The listing builds one solid part. Answer for the finished solid, in the listing's coordinates (mm). Face numbers are marked on the shaded views. A direction names the side the tool comes from. Coordinates: 2 decimals unless noted, no trailing zeros. Loops run counter-clockwise (first coordinate to the right, second up) from the corner with the lowest first, then second, coordinate; pieces in that order, holes last. Notation, with made-up numbers: (33.5, 7) - (92.5, 7) arc R24 ccw to (92.5, 30) - close; hole circle Ø2 at (-39, 62). An arc over 180 degrees is marked (long way). One line per question, with ' | ' between items.
from build123d import *

# Parameters (mm, degrees)
SKETCH_1_W          = 40
SKETCH_1_H          = 30
EXTRUDE_2_DEPTH     = 6
SKETCH_2_W          = 30
SKETCH_2_H          = 8.15479
EXTRUDE_4_DEPTH     = 30
SKETCH_4_R          = 5
CUT_EXTRUDE_1_DEPTH = 51.950956811
FILLET_1_R          = 10
FILLET_2_R          = 10


with BuildPart() as part:
    # Эскиз1 → Бобышка-Вытянуть2 (new body)
    with BuildSketch(Plane.XY):
        Rectangle(SKETCH_1_W, SKETCH_1_H)
    extrude(amount=EXTRUDE_2_DEPTH)

    # Эскиз2 → Бобышка-Вытянуть4 (add)
    with BuildSketch(Plane.XY.offset(6)):
        with Locations((0, -10.922605)):
            Rectangle(SKETCH_2_W, SKETCH_2_H)
    extrude(amount=EXTRUDE_4_DEPTH)

    # Эскиз4 → Вырез-Вытянуть1 (cut, through all)
    with BuildSketch(Plane(origin=(0, -15, 0), x_dir=(-1, 0, 0), z_dir=(0, -1, 0))):
        with Locations(Location((0, -21, 0), (0, 0, 180))):
            Circle(SKETCH_4_R)
    extrude(amount=-CUT_EXTRUDE_1_DEPTH, mode=Mode.SUBTRACT)

    # Скругление1
    fillet_1_edges = [part.edges().sort_by_distance(p)[0] for p in [
        (-15, -10.922605, 36),
    ]]
    fillet(fillet_1_edges, radius=FILLET_1_R)

    # Скругление2
    fillet_2_edges = [part.edges().sort_by_distance(p)[0] for p in [
        (15, -10.922605, 36),
    ]]
    fillet(fillet_2_edges, radius=FILLET_2_R)


solid = part.part
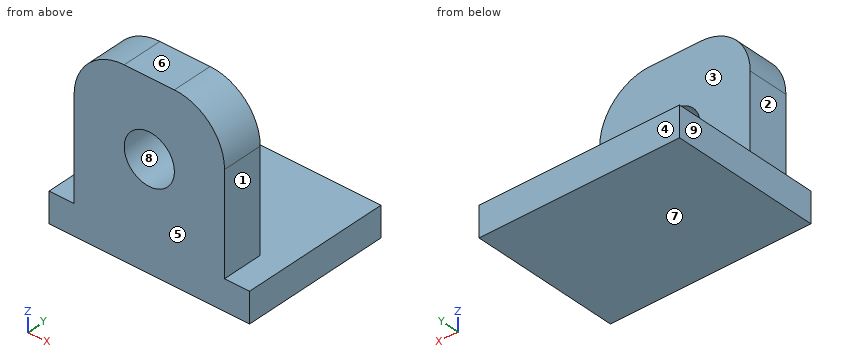
Item 1: Each of these flat-tipped pins is pushed along its axis until it touches: pin 1 Ø4 at (x, z) = (-5, 24.5) entering from +Y; pin 2 Ø3 at (x, y) = (12, 4) entering from +Z; pin 3 Ø9 at (y, z) = (-11.5, 12.5) entering from +X. Where does it stop, or does it pass through?
Taken from the geometry:
pin 1: stops at y = -6.85 | pin 2: stops at z = 6 | pin 3: stops at x = 15
Item 2: The mould has two halves that part along Z. Classify the marked faces 6, 7, 8 and 9: pulls with the +Z half, pulls with the -Z half, needs draft (parallel to the pull), parting line crosses it, or undercut.
Taken from the geometry:
face 6: pulls with the +Z half | face 7: pulls with the -Z half | face 8: undercut | face 9: needs draft
Item 3: Find section A-A, the plane y = -10.5. Write down the section's boundary in (x, z), plus the area to 3 significant figures.
Taken from the geometry:
outline: (-20, 0) - (20, 0) - (20, 6) - (15, 6) - (15, 26) arc R10 ccw to (5, 36) - (-5, 36) arc R10 ccw to (-15, 26) - (-15, 6) - (-20, 6) - close; hole circle Ø10 at (0, 21) | area: 1,020 mm2
Item 4: Find the intervals of material crossed by line 1 (Z direction, x = 0, y = -12); line 2 (Y direction, x = 6, z = 28); line 3 (Z direction, x = 2, y = 6.5), in increasing order. Write a range as [from, to].
Taken from the geometry:
line 1: z = [0, 16], [26, 36] | line 2: y = [-15, -6.85] | line 3: z = [0, 6]
Item 5: Find section D-D, the plane z = 9.5. Write down the section's boundary in (x, y).
Taken from the geometry:
outline: (-15, -15) - (15, -15) - (15, -6.85) - (-15, -6.85) - close
Item 6: Which of the six approach directions +Z, -Z, +X, -X, +Y, -Y give full straight-line access (tool end or side, diameter ignored) to the marked faces 1, 2, 3, 4 and 5?
Taken from the geometry:
face 1: +Z, +X, +Y, -Y | face 2: +Z, -X, +Y, -Y | face 3: +Z, +X, -X, +Y | face 4: +Z, -Z, +X, -X, +Y | face 5: +Z, -Z, +X, -X, -Y
Item 7: Find section C-C, the plane z = 21. Write down the section's boundary in (x, y).
Taken from the geometry:
outline: (-15, -15) - (-5, -15) - (-5, -6.85) - (-15, -6.85) - close; (5, -15) - (15, -15) - (15, -6.85) - (5, -6.85) - close
Item 8: Find section B-B, the plane x = 0. Write down the section's boundary in (y, z).
Taken from the geometry:
outline: (-15, 0) - (15, 0) - (15, 6) - (-6.85, 6) - (-6.85, 16) - (-15, 16) - close; (-15, 26) - (-6.85, 26) - (-6.85, 36) - (-15, 36) - close
